from build123d import *

# Parameters (mm, degrees)
SHOULDER_START    = 7
PROFILE_1_R       = 4
SHOULDER_DEPTH    = 12
M6_THREAD_START   = -4
PROFILE_2_R       = 3
M6_THREAD_DEPTH   = 11
SOCKET_HEAD_START = 19
PROFILE_3_R       = 6.5
SOCKET_HEAD_DEPTH = 5.5


with BuildPart() as part:
    # Profile_1 → Shoulder (new body)
    with BuildSketch(Plane.XY.offset(SHOULDER_START)):
        Circle(PROFILE_1_R)
    extrude(amount=SHOULDER_DEPTH)

    # Profile_2 → M6_thread (add)
    with BuildSketch(Plane.XY.offset(M6_THREAD_START)):
        Circle(PROFILE_2_R)
    extrude(amount=M6_THREAD_DEPTH)

    # Profile_3 → Socket_head (add)
    with BuildSketch(Plane.XY.offset(SOCKET_HEAD_START)):
        Circle(PROFILE_3_R)
        Polygon((2, 1.154700538), (0, 2.309401077), (-2, 1.154700538), (-2, -1.154700538), (0, -2.309401077), (2, -1.154700538), align=None, mode=Mode.SUBTRACT)
    extrude(amount=SOCKET_HEAD_DEPTH)


solid = part.part
Work out the finished part from the listing and answer in its coordinate system (mm). A direction names the side the tool comes from. Give positions to 0.01 mm unless a question says otherwise; leave off trailing zeros. Order: outer loops, then holes, each group sorted by start corner. A loop starts at its lowest first (then second) coordinate and runs counter-clockwise, first axis right, second up. Notation, with made-up numbers: (-38, -17) -> (-32, -17) arc R14 cw to (-32, 6) -> close; hole circle Ø10 at (-39, 23). An arc over 180 degrees is marked (long way). One line per item, written item: value.
Item 1: Find section C-C, the plane z = 4.75. Give the vertices of the cut face in (x, y).
Answer sheet:
outline: circle Ø6 at (0, 0)
Item 2: Flat-ended cylindrical pins translate along their axes: P1, Ø3, axis at y = 0, z = 11.5, coming from the -X side; P2, Ø1.5, axis at x = 2.5, z = 18.5, coming from the +Y side; P3, Ø6, axis at y = 1, z = 0, coming from the +X side. Find the tip coordinate at first contact, or state that the pin passes through.
Answer sheet:
P1: x = -4
P2: y = 6.2
P3: x = 3
Item 3: Find section D-D, the plane x = -4.5. Give the vertices of the cut face in (y, z).
Answer sheet:
outline: (-4.69, 19) -> (4.69, 19) -> (4.69, 24.5) -> (-4.69, 24.5) -> close
Item 4: Find section A-A, the plane y = 0. Give the vertices of the cut face in (x, z).
Answer sheet:
outline: (-6.5, 19) -> (-4, 19) -> (-4, 7) -> (-3, 7) -> (-3, -4) -> (3, -4) -> (3, 7) -> (4, 7) -> (4, 19) -> (6.5, 19) -> (6.5, 24.5) -> (2, 24.5) -> (2, 19) -> (-2, 19) -> (-2, 24.5) -> (-6.5, 24.5) -> close
Item 5: Find section B-B, the plane z = 20.75. Give the vertices of the cut face in (x, y).
Answer sheet:
outline: circle Ø13 at (0, 0); hole (-2, -1.15) -> (0, -2.31) -> (2, -1.15) -> (2, 1.15) -> (0, 2.31) -> (-2, 1.15) -> close
Item 6: Determine the mould class of faces 1 (the cylindrical face through (-5.158, -3.955, 21.712)), 2 (the flat face through (-1.014, -1.724, 21.712)), 3 (the flat face through (1, 3, 7)) for opening direction X: released by +X, released by -X, zero draft, split by the parting line, or undercut.
Answer sheet:
face 1: split by the parting line
face 2: undercut
face 3: zero draft
Item 7: A tool of negligible diameter and unlimited length cuts with its end or side. For faces 4 (the flat face through (0, 0, -4)), 5 (the flat face through (-0.99, 1.74, 21.71)), 6 (the cylindrical face through (-0.867, -3.905, 12.916)), from which of +Z, -Z, +X, -X, +Y, -Y can it reach the whole face along a straight path? Write none if from no direction.
Answer sheet:
face 4: -Z, +X, -X, +Y, -Y
face 5: +Z
face 6: -Z
Item 8: Straight lines are drawn through the part: probe 1 along Z at (x, y) = (-1.25, -4); probe 2 along Z at (x, y) = (-1.5, 3.5); probe 3 along Y at (x, z) = (0, 17). For each, find the intervals that lie inside material, in ascending order.
Answer sheet:
probe 1: 19 to 24.5
probe 2: 7 to 24.5
probe 3: -4 to 4
